```python
from build123d import *

# Parameters (mm, degrees)
SKETCH_1_R          = 14
SKETCH_1_R_2        = 1.5
EXTRUDE_1_DEPTH     = 4
SKETCH_2_R          = 7.5
EXTRUDE_2_DEPTH     = 12
SKETCH_3_R          = 3
CUT_EXTRUDE_1_DEPTH = 17
FILLET_1_R          = 0.5
FILLET_2_R          = 0.5
SKETCH_4_R          = 2
CUT_EXTRUDE_3_DEPTH = 15.0000001


with BuildPart() as part:
    # 草图1 → 凸台-拉伸1 (new body)
    with BuildSketch(Plane.XY):
        Circle(SKETCH_1_R)
        with Locations((0, 11.5)):
            Circle(SKETCH_1_R_2, mode=Mode.SUBTRACT)
        with Locations((9.959292144, 5.75)):
            Circle(SKETCH_1_R_2, mode=Mode.SUBTRACT)
        with Locations((9.959292144, -5.75)):
            Circle(SKETCH_1_R_2, mode=Mode.SUBTRACT)
        with Locations((0, -11.5)):
            Circle(SKETCH_1_R_2, mode=Mode.SUBTRACT)
        with Locations((-9.959292144, -5.75)):
            Circle(SKETCH_1_R_2, mode=Mode.SUBTRACT)
        with Locations((-9.959292144, 5.75)):
            Circle(SKETCH_1_R_2, mode=Mode.SUBTRACT)
    extrude(amount=EXTRUDE_1_DEPTH)

    # 草图2 → 凸台-拉伸2 (add)
    with BuildSketch(Plane.XY.offset(4)):
        Circle(SKETCH_2_R)
    extrude(amount=EXTRUDE_2_DEPTH)

    # 草图3 → 切除-拉伸1 (cut, through all)
    with BuildSketch(Plane.XY.offset(16)):
        Circle(SKETCH_3_R)
    extrude(amount=-CUT_EXTRUDE_1_DEPTH, mode=Mode.SUBTRACT)

    # 圆角1
    fillet_1_edges = [part.edges().sort_by_distance(p)[0] for p in [
        (-14, 0, 0),
        (-14, 0, 4),
    ]]
    fillet(fillet_1_edges, radius=FILLET_1_R)

    # 圆角2
    fillet_2_edges = [part.edges().sort_by_distance(p)[0] for p in [
        (-7.5, 0, 4),
    ]]
    fillet(fillet_2_edges, radius=FILLET_2_R)

    # 草图4 → 切除-拉伸3 (cut, through all)
    with BuildSketch(Plane(origin=(0, 0, 0), x_dir=(1, 0, 0), z_dir=(0, 1, 0))):
        with Locations((0, -9.370984313)):
            Circle(SKETCH_4_R)
    extrude(amount=CUT_EXTRUDE_3_DEPTH, mode=Mode.SUBTRACT)


solid = part.part
```
Input: part model. Units: mm. Frame: model coordinates. A direction names the side the tool comes from. Coordinates: 2 decimals unless noted, no trailing zeros. Loops run counter-clockwise (first coordinate to the right, second up) from the corner with the lowest first, then second, coordinate; pieces in that order, holes last. Notation, with made-up numbers: M 87.5,-9 L 125.5,-9 A26 ccw 125.5,10 Z; hole C 24,40.25 d8. An arc over 180 degrees is marked long. Answer in a Markdown table with one row per item.
1. Material intervals for line 1 (Y direction, x = 0, z = 0.85); line 2 (X direction, y = -6.75, z = 2); line 3 (Z direction, x = 9.5, y = 9.5), sorted ascending.
Response:
| item | result |
|---|---|
| line 1 | y = -14 to -13, -10 to -3, 3 to 10, 13 to 14 |
| line 2 | x = -12.27 to -11.08, -8.84 to 8.84, 11.08 to 12.27 |
| line 3 | z = 0 to 4 |
2. Section A-A, the plane x = 0. Count the separate pieces of the cut face and the enclosed holes in it, then the cut area to 3 significant figures.
Response:
| item | result |
|---|---|
| separate pieces | 5 |
| enclosed holes | 0 |
| area | 154 mm2 |
3. First-contact query: pin 1 (2 mm diameter, centred on x = -10.5, y = 0, fed in from -Z); pin 2 (3.5 mm diameter, centred on x = 0, y = -11.5, fed in from +Z); pin 3 (6 mm diameter, centred on y = 0, z = 8, fed in from +X); pin 4 (5 mm diameter, centred on x = 0, z = 9.37, fed in from -Y). Flat tips, straight axial feed; report the tip coordinate or a pass-through.
Response:
| item | result |
|---|---|
| pin 1 | stops at z = 0 |
| pin 2 | stops at z = 4 |
| pin 3 | stops at x = 7.5 |
| pin 4 | stops at y = -7.5 |
4. Draft query along Y for faces 4 (the cylindrical face through (-8.57, -6.32, 1.97)), 5 (the cylindrical face through (-1.63, -7.32, 10.17)), 6 (the flat face through (3.2, 0.1, 16)). Return one class per face: pulls with the +Y half, pulls with the -Y half, needs draft (parallel to the pull), parting line crosses it, or undercut.
Response:
| item | result |
|---|---|
| face 4 | undercut |
| face 5 | parting line crosses it |
| face 6 | needs draft |
5. Reachability of faces 1 (the cylindrical face through (0, 10, 2)), 2 (the flat face through (6, -6, 4)), 3 (the cylindrical face through (1.908, 4.835, 8.77)) from +Z, -Z, +X, -X, +Y, -Y: full face, straight path, thin tool, end or side. Return the list, or none.
Response:
| item | result |
|---|---|
| face 1 | +Z, -Z |
| face 2 | +Z |
| face 3 | +Y |
6. Section B-B, the plane z = 6. Output: boundary loops of the cut face in (x, y).
Response:
| item | result |
|---|---|
| outline | C 0,0 d15; hole C 0,0 d6 |
